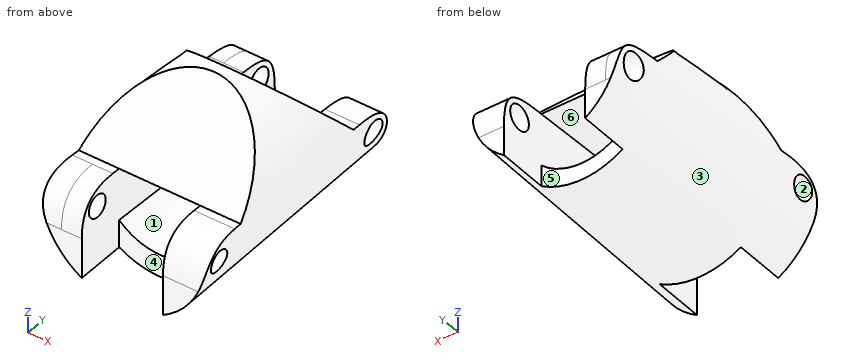
```python
from build123d import *

# Parameters (mm, degrees)
SKETCH1_R                     = 10
BOSS_EXTRUDE1_DEPTH           = 25
BOSS_EXTRUDE1_TAPER           = 2
BOSS_EXTRUDE1_OTHER_WAY_DEPTH = 6
BOSS_EXTRUDE1_OTHER_WAY_TAPER = -2
CUT_EXTRUDE1_DEPTH            = 29.86985947
CUT_EXTRUDE1_DEPTH_BACK       = 29.86985947
SKETCH3_W                     = 10
SKETCH3_H                     = 6
CUT_EXTRUDE2_DEPTH            = 25
CUT_EXTRUDE3_DEPTH            = 31.99296746
CUT_EXTRUDE3_DEPTH_BACK       = 31.99296746
SKETCH4_R                     = 1.5
FILLET2_SIZE                  = 5
CUT_EXTRUDE5_DEPTH            = 29.869859627
CUT_EXTRUDE5_DEPTH_BACK       = 29.869859627
SKETCH8_W                     = 10
SKETCH8_H                     = 6
CUT_EXTRUDE6_DEPTH            = 30.190018507
CUT_EXTRUDE7_DEPTH            = 29.796430368
CUT_EXTRUDE8_DEPTH            = 31.924580015
CUT_EXTRUDE8_DEPTH_BACK       = 31.924580015
SKETCH9_R                     = 1.351518808
FILLET3_SIZE                  = 5


with BuildPart() as part:
    # Sketch1 → Boss-Extrude1 (new body)
    with BuildSketch(Plane(origin=(0, 0, 0), x_dir=(1, 0, 0), z_dir=(0, 1, 0))):
        Circle(SKETCH1_R)
    extrude(amount=BOSS_EXTRUDE1_DEPTH, taper=BOSS_EXTRUDE1_TAPER)

    # Sketch1 → Boss-Extrude1 other way (add)
    with BuildSketch(Plane(origin=(0, 0, 0), x_dir=(1, 0, 0), z_dir=(0, 1, 0))):
        Circle(SKETCH1_R)
    extrude(amount=-BOSS_EXTRUDE1_OTHER_WAY_DEPTH, taper=BOSS_EXTRUDE1_OTHER_WAY_TAPER)

    # Sketch2 → Cut-Extrude1 (cut, two sides: drawn at the far end of the back side and taken through both)
    with BuildSketch(Plane(origin=(0, 0, 0), x_dir=(0, 0, -1), z_dir=(1, 0, 0)).offset(-CUT_EXTRUDE1_DEPTH_BACK)):
        Polygon((-0.873019237, 25), (-0.873019237, 19), (-12.898136563, 6.974882674), (-12.898136563, 25), align=None)
    extrude(amount=CUT_EXTRUDE1_DEPTH + CUT_EXTRUDE1_DEPTH_BACK, mode=Mode.SUBTRACT)

    # Sketch3 → Cut-Extrude2 (cut)
    with BuildSketch(Plane.XY.offset(0.873019237)):
        with Locations((0, 22)):
            Rectangle(SKETCH3_W, SKETCH3_H)
    extrude(amount=-CUT_EXTRUDE2_DEPTH, mode=Mode.SUBTRACT)

    # Sketch4 → Cut-Extrude3 (cut, two sides: drawn at the far end of the back side and taken through both)
    with BuildSketch(Plane(origin=(-5, 0, 0), x_dir=(0, 0, -1), z_dir=(1, 0, 0)).offset(-CUT_EXTRUDE3_DEPTH_BACK)):
        with Locations(Location((1.626980763, 22.5, 0), (0, 0, 90))):
            Circle(SKETCH4_R)
    extrude(amount=CUT_EXTRUDE3_DEPTH + CUT_EXTRUDE3_DEPTH_BACK, mode=Mode.SUBTRACT)

    # Fillet2
    # a fillet whose section is not a circle: 5 mm, written as the material it takes off along each edge
    with BuildSketch(Plane(origin=(-7.5, 25, 0.873019237), x_dir=(0, -1, 0), z_dir=(1, 0, 0))) as fillet2_piece_1:
        with BuildLine():
            Bezier((FILLET2_SIZE, 0), (0, 0), (0, FILLET2_SIZE), weights=[1, 1.5, 1])
            Line((0, FILLET2_SIZE), (0, 0))
            Line((0, 0), (FILLET2_SIZE, 0))
        make_face()
    extrude(amount=29.085131549, mode=Mode.SUBTRACT)
    with BuildSketch(Plane(origin=(-21.585131549, 25, 0.873019237), x_dir=(0, 0, -1), z_dir=(1, 0, 0))) as fillet2_piece_2:
        with BuildLine():
            Bezier((FILLET2_SIZE, 0), (0, 0), (0, -FILLET2_SIZE), weights=[1, 1.5, 1])
            Line((0, -FILLET2_SIZE), (0, 0))
            Line((0, 0), (FILLET2_SIZE, 0))
        make_face()
    extrude(amount=29.085131549, mode=Mode.SUBTRACT)

    # Sketch7 → Cut-Extrude5 (cut, two sides: drawn at the far end of the back side and taken through both)
    with BuildSketch(Plane(origin=(0, 0, 0), x_dir=(0, 0, -1), z_dir=(1, 0, 0)).offset(-CUT_EXTRUDE5_DEPTH_BACK)):
        Polygon((-0.873019237, -6), (-0.873019237, 0), (-11.31781305, 10.444793812), (-11.31781305, -6), align=None)
    extrude(amount=CUT_EXTRUDE5_DEPTH + CUT_EXTRUDE5_DEPTH_BACK, mode=Mode.SUBTRACT)

    # Sketch8 → Cut-Extrude6 (cut, through all)
    with BuildSketch(Plane.XY.offset(0.873019237)):
        with Locations((0, -3)):
            Rectangle(SKETCH8_W, SKETCH8_H)
    extrude(amount=-CUT_EXTRUDE6_DEPTH, mode=Mode.SUBTRACT)

    # Sketch6 → Cut-Extrude7 (cut, through all)
    with BuildSketch(Plane(origin=(0, 19, 0), x_dir=(1, 0, 0), z_dir=(0, 1, 0))):
        with BuildLine():
            Line((5, 5.368827729), (5, -0.873019237))
            Line((5, -0.873019237), (-5, -0.873019237))
            Line((-5, -0.873019237), (-5, 5.368827729))
            ThreePointArc((-5, 5.368827729), (0, 7.33650538), (5, 5.368827729))
        make_face()
    extrude(amount=-CUT_EXTRUDE7_DEPTH, mode=Mode.SUBTRACT)

    # Sketch9 → Cut-Extrude8 (cut, two sides: drawn at the far end of the back side and taken through both)
    with BuildSketch(Plane(origin=(-5, 0, 0), x_dir=(0, 0, -1), z_dir=(1, 0, 0)).offset(-CUT_EXTRUDE8_DEPTH_BACK)):
        with Locations(Location((1.626980763, -3.5, 0), (0, 0, 90))):
            Circle(SKETCH9_R)
    extrude(amount=CUT_EXTRUDE8_DEPTH + CUT_EXTRUDE8_DEPTH_BACK, mode=Mode.SUBTRACT)

    # Fillet3
    # a fillet whose section is not a circle: 5 mm, written as the material it takes off along each edge
    with BuildSketch(Plane(origin=(22.672130078, -6, 0.873019237), x_dir=(0, 0, -1), z_dir=(-1, 0, 0))) as fillet3_piece_1:
        with BuildLine():
            Bezier((FILLET3_SIZE, 0), (0, 0), (0, -FILLET3_SIZE), weights=[1, 1, 1])
            Line((0, -FILLET3_SIZE), (0, 0))
            Line((0, 0), (FILLET3_SIZE, 0))
        make_face()
    extrude(amount=30.172130078, mode=Mode.SUBTRACT)
    with BuildSketch(Plane(origin=(7.5, -6, 0.873019237), x_dir=(0, 1, 0), z_dir=(-1, 0, 0))) as fillet3_piece_2:
        with BuildLine():
            Bezier((FILLET3_SIZE, 0), (0, 0), (0, FILLET3_SIZE), weights=[1, 1, 1])
            Line((0, FILLET3_SIZE), (0, 0))
            Line((0, 0), (FILLET3_SIZE, 0))
        make_face()
    extrude(amount=30.172130078, mode=Mode.SUBTRACT)


solid = part.part
```
Check sheet for the modelled part. Datum: model origin and axes. Units: mm. Face numbers are marked on the shaded views. A direction names the side the tool comes from. Round coordinates to 2 decimals unless told otherwise and drop trailing zeros. Write each loop counter-clockwise with the first axis right and the second up, starting at its lowest first coordinate (ties: lowest second). Pieces come first, ordered by that corner, then holes. Notation, with made-up numbers: (41.25, 80) -> (97.25, 80) arc R24 cw to (97.25, 96) -> close; hole circle Ø4 at (65.25, 66). An arc over 180 degrees is marked (long way). Put each result on its own line as item: value.
(1) Sectioned sample at B-B (y = 12.5). Enter the section's corners in (x, z).
Values found:
outline: (-6.09, 7.37) arc R9.56 ccw (long way) to (6.09, 7.37) -> close; hole (-5, -5.37) arc R7.34 ccw to (5, -5.37) -> (5, 0.87) -> (-5, 0.87) -> close
(2) Mould release check, pull along X, two halves, no side actions. Record for the marked faces 1, 2 and 3: released by +X, released by -X, zero draft, split by the parting line, or undercut.
Values found:
face 1: undercut
face 2: zero draft
face 3: split by the parting line
(3) Go/stop test with flat-tipped pins: pin 1 Ø1.5 at (x, z) = (-2.5, 4.5) entering from +Y; pin 2 Ø3 at (y, z) = (7.5, -2.5) entering from -X; pin 3 Ø1.1 at (x, y) = (-6.5, -0.5) entering from +Z; pin 4 Ø10 at (x, z) = (5.5, -2) entering from -Y. Record where each tip stops, or that it passes through.
Values found:
pin 1: stops at y = 16.12
pin 2: stops at x = -9.7
pin 3: stops at z = 0.92
pin 4: stops at y = -6
(4) Material ranges on line 1 (Y direction, x = 6.5, z = -2.75); line 2 (X direction, y = -2.5, z = -4); line 3 (Y direction, x = 6, z = -1.5), recorded low to high.
Values found:
line 1: y = -5.89 to -4.25, -2.75 to 21.51, 23.49 to 24.95
line 2: x = -9.26 to -5, 5 to 9.26
line 3: y = -5.52 to -4.85, -2.15 to 21.01, 23.99 to 24.74
(5) Tool access check on the marked faces 4, 5 and 6. Record the directions out of +Z, -Z, +X, -X, +Y, -Y that give a thin tool (end or side, any length) a straight path to the whole face; none if there is none.
Values found:
face 4: +Z, -Z, -Y
face 5: +Z, -Z, +Y
face 6: +Y, -Y
(6) Sectioned sample at A-A (x = 0). Enter the section's corners in (y, z), plus the area to 3 significant figures.
Values found:
outline: (0, -10) -> (19, -9.34) -> (19, -7.34) -> (0, -7.34) -> close; (0, 0.87) -> (19, 0.87) -> (10.23, 9.64) -> (8.82, 9.69) -> close
area: 134 mm^2
(7) Sectioned sample at C-C (z = -1). Count the separate pieces of the cut face and the enclosed holes in it, plus the area to 3 significant figures.
Values found:
separate pieces: 6
enclosed holes: 0
area: 228 mm^2
